```python
from build123d import *

# Parameters (mm, degrees)
SKETCH1_W           = 38.1
SKETCH1_H           = 21.59
BOSS_EXTRUDE1_DEPTH = 3.81
SKETCH2_W           = 3.81
SKETCH2_H           = 21.59
BOSS_EXTRUDE2_DEPTH = 38.1
FILLET1_R           = 5.08
FILLET2_R           = 3.81
SKETCH4_R           = 3.048
BOSS_EXTRUDE3_DEPTH = 2.54
SKETCH5_R           = 3.048
BOSS_EXTRUDE4_DEPTH = 2.54
FILLET3_R           = 2.54


# Some blends are built 0.0001 mm under size
with BuildPart() as part:
    # Sketch1 → Boss-Extrude1 (new body)
    with BuildSketch(Plane(origin=(0, 0, 0), x_dir=(1, 0, 0), z_dir=(0, 1, 0))):
        with Locations((-28.525509612, -11.453306042)):
            Rectangle(SKETCH1_W, SKETCH1_H)
    extrude(amount=BOSS_EXTRUDE1_DEPTH)

    # Sketch2 → Boss-Extrude2 (add)
    with BuildSketch(Plane(origin=(0, 3.81, 0), x_dir=(1, 0, 0), z_dir=(0, 1, 0))):
        with Locations((-45.670509612, -11.453306042)):
            Rectangle(SKETCH2_W, SKETCH2_H)
    extrude(amount=BOSS_EXTRUDE2_DEPTH)

    # Fillet1
    # the kernel refuses this fillet: 5.08 mm, written as the material it adds along each edge
    with BuildSketch(Plane(origin=(-43.765509612, 3.81, 0.658306042), x_dir=(1, 0, 0), z_dir=(0, 0, 1))) as fillet1_piece_1:
        with BuildLine():
            CenterArc((FILLET1_R, FILLET1_R), FILLET1_R, 180, 90)
            Line((0, FILLET1_R), (0, 0))
            Line((0, 0), (FILLET1_R, 0))
        make_face()
    extrude(amount=21.59)
    # the kernel refuses this fillet: 5.08 mm, written as the material it takes off along each edge
    with BuildSketch(Plane(origin=(-9.475509612, 3.81, -11.638416082), x_dir=(-1, 0, 0), z_dir=(0, 0, 1))) as fillet1_2_piece_1:
        with BuildLine():
            CenterArc((4.91868885, 5.08), FILLET1_R, 194.477512186, 75.522487814)
            Line((0, 3.81), (0, 0))
            Line((0, 0), (4.91868885, 0))
        make_face()
    extrude(amount=46.183444248, mode=Mode.SUBTRACT)
    with BuildSketch(Plane(origin=(-43.765509612, 41.91, -11.638416082), x_dir=(-1, 0, 0), z_dir=(0, 0, 1))) as fillet1_2_piece_2:
        with BuildLine():
            CenterArc((5.08, 4.91868885), FILLET1_R, 180, 75.522487814)
            Line((0, 4.91868885), (0, 0))
            Line((0, 0), (3.81, 0))
        make_face()
    extrude(amount=46.183444248, mode=Mode.SUBTRACT)

    # Fillet2
    fillet2_edges = [part.edges().sort_by_distance(p)[0] for p in [
        (-47.575509612, 0, 11.453306042),
    ]]
    fillet(fillet2_edges, radius=FILLET2_R)

    # Sketch4 → Boss-Extrude3 (add)
    with BuildSketch(Plane(origin=(-43.765509612, 0, 0), x_dir=(0, 0, -1), z_dir=(1, 0, 0))):
        with Locations(Location((-11.392673718, 29.655405516, 0), (0, 0, 180))):
            Circle(SKETCH4_R)
        with Locations(Location((-11.252567749, 17.758913463, 0), (0, 0, 180))):
            Circle(SKETCH4_R)
    extrude(amount=BOSS_EXTRUDE3_DEPTH)

    # Sketch5 → Boss-Extrude4 (add)
    with BuildSketch(Plane(origin=(0, 3.81, 0), x_dir=(1, 0, 0), z_dir=(0, 1, 0))):
        with Locations(Location((-32.655326175, -11.503425175, 0), (0, 0, 90))):
            Circle(SKETCH5_R)
        with Locations(Location((-21.629116904, -11.443282215, 0), (0, 0, 90))):
            Circle(SKETCH5_R)
    extrude(amount=BOSS_EXTRUDE4_DEPTH)

    # Fillet3
    fillet3_edges = [part.edges().sort_by_distance(p)[0] for p in [
        (-41.225509612, 29.655405516, 8.344673718),
        (-41.225509612, 17.758913463, 8.204567749),
        (-32.655326175, 6.35, 14.551425175),
        (-21.629116904, 6.35, 14.491282215),
    ]]
    fillet(fillet3_edges, radius=FILLET3_R - 0.0001)  # a hair under: the kernel refuses the full size


solid = part.part
```
Work out the finished part from the listing and answer in its coordinate system (mm). A direction names the side the tool comes from. Round coordinates to 2 decimals unless told otherwise and drop trailing zeros. Loops run counter-clockwise (first coordinate to the right, second up) from the corner with the lowest first, then second, coordinate; pieces in that order, holes last.
(1) The mould has two halves that part along Y. Classify faces 4 (the flat face through (-44, 13, 22.248)), 5 (the cylindrical face through (-44.801, 40.065, 11.302)), 6 (the flat face through (-43.766, 23, 12)): pulls with the +Y half, pulls with the -Y half, needs draft (parallel to the pull), parting line crosses it, or undercut.
Computed values:
face 4: needs draft
face 5: pulls with the +Y half
face 6: undercut
(2) The part is cut by section A-A, the plane z = 4.75. Give the vertices of the cut face in (x, y), and give its area (3 significant figures).
Computed values:
outline: (-47.58, 3.81) arc R3.81 ccw to (-43.77, 0) - (-9.48, 0) arc R5.08 ccw to (-14.39, 3.81) - (-38.69, 3.81) arc R5.08 cw to (-43.77, 8.89) - (-43.77, 36.99) arc R5.08 ccw to (-47.58, 41.91) - close
area: 283 mm2
(3) The part is cut by section B-B, the plane x = -28. Give the vertices of the cut face in (y, z), and give its area (3 significant figures).
Computed values:
outline: (0, 0.66) - (3.81, 0.66) - (3.81, 22.25) - (0, 22.25) - close
area: 82.3 mm2
(4) Find the intervals of material crossed by L1, parallel to X at y = 21.5, z = 15; L2, parallel to Y at x = -39, z = 4.25; L3, parallel to X at y = 31, z = 9.75, in increasing order.
Computed values:
L1: x = -47.58 to -43.77
L2: y = 0 to 3.82
L3: x = -47.58 to -41.8
(5) For faces 1 (the cylindrical face through (-42.32, 5.34, 11.3)), 2 (the flat face through (-27, 3.81, 11)), 3 (the flat face through (-21.6, 6.35, 11.5)), determine the directions among +Z, -Z, +X, -X, +Y, -Y from which every point of the face is accessible in a straight line to the end or side of a thin tool.
Computed values:
face 1: +Z, -Z
face 2: +Y
face 3: +Z, -Z, +X, +Y
(6) The part is cut by section C-C, the plane y = 36. Give the vertices of the cut face in (x, z), and give its area (3 significant figures).
Computed values:
outline: (-47.58, 0.66) - (-43.77, 0.66) - (-43.77, 22.25) - (-47.58, 22.25) - close
area: 82.3 mm2
(7) The part is cut by section D-D, the plane x = -43. Give the number of separate pieces and of enclosed holes in the cut face, and give its area (3 significant figures).
Computed values:
separate pieces: 3
enclosed holes: 0
area: 188 mm2
(8) Each of these flat-tipped pins is pushed along its axis until it touches: P1, Ø0.5, axis at x = -32.5, z = 11.5, coming from the +Y side; P2, Ø3, axis at x = -25, z = 6.5, coming from the +Y side; P3, Ø1, axis at y = 11.5, z = 11, coming from the +X side. Where does it stop, or does it pass through?
Computed values:
P1: stops at y = 6.35
P2: stops at y = 3.81
P3: stops at x = -43.77
